Autodesk Inventor part; units mm, degrees
ref_plane "YZ Plane" through (0, 0, 0) normal (1, 0, 0) x (0, 1, 0)
ref_plane "XZ Plane" through (0, 0, 0) normal (0, 1, 0) x (-1, 0, 0)
ref_plane "XY Plane" through (0, 0, 0) normal (0, 0, 1) x (1, 0, 0)
sketch "Sketch1" plane through (0, 0, 0) normal (0, 1, 0) x (-1, 0, 0)
  line L0 (85, 50) -> (-85, 50)
  line L1 (-85, 50) -> (-85, -50)
  line L2 (-85, -50) -> (85, -50)
  line L3 (85, -50) -> (85, 50)
  line L4 (85, 50) -> (-85, -50) construction
  line L5 (-85, 50) -> (85, -50) construction
  point P0 (0, 0)
  dimension "d0" = 170
  dimension "d1" = 100
extrude "Extrusion1" add sketch "Sketch1" along normal blind 3.125
sketch "Sketch2" plane through (0, 3.125, 0) normal (0, 1, 0) x (1, 0, 0)
  line L0 (-26.702, 10) -> (-6.702, 10)
  line L1 (-6.702, 10) -> (-6.702, -10)
  line L2 (-6.702, -10) -> (-26.702, -10)
  line L3 (-26.702, -10) -> (-26.702, 10)
  line L4 (-26.702, 10) -> (-6.702, -10) construction
  line L5 (-6.702, 10) -> (-26.702, -10) construction
  circle A0 centre (-16.702, 0) radius 7.5
  line L6 (25.8262, 10) -> (45.8262, 10)
  line L7 (45.8262, 10) -> (45.8262, -10)
  line L8 (45.8262, -10) -> (25.8262, -10)
  line L9 (25.8262, -10) -> (25.8262, 10)
  line L10 (25.8262, 10) -> (45.8262, -10) construction
  line L11 (45.8262, 10) -> (25.8262, -10) construction
  circle A1 centre (35.8262, 0) radius 7.5
  line L12 (0.1504, 0) -> (2.6516, 0) construction
  point P0 (0, 0)
  dimension "d13" = 0
  dimension "d4" = 20
  dimension "d5" = 20
  dimension "d6" = 15
  dimension "d14" = 20
  dimension "d15" = 20
  dimension "d16" = 15
extrude "Extrusion2" add sketch "Sketch2" along normal blind 22.4 contours A0 | A1
extrude "Extrusion3" add sketch "Sketch2" along normal blind 10 contours L0 L1 L2 L3 | L6 L7 L8 L9 | A1
sketch "Sketch3" plane through (-16.702, 25.525, 0) normal (0, 1, 0) x (1, 0, 0)
  circle A0 centre (0, 0) radius 3
  point P0 (16.702, 0)
  dimension "d11" = 6
extrude "Extrusion4" cut sketch "Sketch3" against normal blind 7
sketch "Sketch4" plane through (35.8262, 25.525, 0) normal (0, 1, 0) x (1, 0, 0)
  circle A0 centre (0, 0) radius 3
  point P0 (-35.8262, 0)
  dimension "d17" = 6
extrude "Extrusion5" cut sketch "Sketch4" against normal blind 7
sketch "Sketch5" plane through (0, 3.125, 0) normal (0, 1, 0) x (1, 0, 0)
  line L0 (85, 50) -> (-85, 50)
  line L1 (-85, 50) -> (85, 50)
  line L2 (85, 50) -> (85, 51.3)
  line L3 (85, 51.3) -> (-85, 51.3)
  line L4 (-85, 51.3) -> (-85, 50)
  line L5 (-85, -50) -> (85, -50)
  line L6 (-85, -50) -> (85, -50)
  line L7 (85, -50) -> (85, -51.3)
  line L8 (85, -51.3) -> (-85, -51.3)
  line L9 (-85, -51.3) -> (-85, -50)
  line L10 (85, -51.3) -> (87, -51.3)
  line L11 (87, -51.3) -> (87, 51.3)
  line L12 (87, 51.3) -> (85, 51.3)
  line L13 (85, 51.3) -> (85, -51.3)
  point P0 (0, 0)
  point P1 (85, -50)
  dimension "d20" = 1.3
  dimension "d21" = 1.3
  dimension "d22" = 2
extrude "Extrusion6" add sketch "Sketch5" along normal blind 25.525
sketch "Sketch6" plane through (-85, 0, 50) normal (0, 0, 1) x (1, 0, 0)
  line L0 (170, 0) -> (0, 0)
  line L1 (170, 0) -> (170, 3.125)
  line L2 (0, 0) -> (170, 0)
  line L3 (170, 0) -> (170, 3.125)
  line L4 (170, 3.125) -> (0, 3.125)
  line L5 (0, 3.125) -> (0, 0)
  point P0 (85, 0)
extrude "Extrusion7" add sketch "Sketch6" along normal blind 1.3
sketch "Sketch7" plane through (85, 0, -50) normal (0, 0, -1) x (-1, 0, 0)
  line L0 (0, 0) -> (0, 3.125)
  line L1 (170, 0) -> (170, 28.65)
  line L2 (0, 0) -> (170, 0)
  line L3 (170, 0) -> (170, 2.2028)
  line L4 (170, 2.2028) -> (0, 2.2028)
  line L5 (0, 2.2028) -> (0, 0)
extrude "Extrusion8" add sketch "Sketch7" along normal blind 1.3
sketch "Sketch8" plane through (85, 0, 51.3) normal (1, 0, 0) x (0, 0, -1)
  line L0 (0, 0) -> (0, 3.125)
  line L1 (0, 0) -> (102.6, 0)
  line L2 (0, 3.125) -> (102.6, 3.125)
  line L3 (102.6, 3.125) -> (102.6, 0)
  line L4 (102.6, 0) -> (0, 0)
  line L5 (0, 0) -> (0, 3.125)
  point P0 (51.3, 0)
extrude "Extrusion9" add sketch "Sketch8" along normal blind 2
sketch "Sketch9" plane through (0, 3.125, 0) normal (0, 1, 0) x (1, 0, 0)
  line L0 (85, -50) -> (85, 50)
  line L1 (85, 50) -> (65, 50)
  line L2 (65, 50) -> (65, 45)
  line L3 (65, 45) -> (85, 45)
  line L4 (85, 45) -> (85, 50)
  line L5 (85, -50) -> (65, -50)
  line L6 (65, -50) -> (65, -45)
  line L7 (65, -45) -> (85, -45)
  line L8 (85, -45) -> (85, -50)
  point P0 (0, 0)
  dimension "d31" = 20
  dimension "d32" = 5
  dimension "d33" = 20
  dimension "d34" = 5
extrude "Extrusion10" add sketch "Sketch9" along normal blind 22.4
sketch "Sketch10" plane through (-85, 3.125, 50) normal (0, 0, -1) x (-1, 0, 0)
  line L0 (-170, 25.525) -> (0, 25.525)
  line L1 (-143.8389, 3.6428) -> (-91.9175, 3.6428)
  line L2 (-91.9175, 3.6428) -> (-91.9175, 25.525)
  line L3 (-91.9175, 25.525) -> (-143.8389, 25.525)
  line L4 (-143.8389, 25.525) -> (-143.8389, 3.6428)
  point P0 (-150, 27.4)
  point P1 (-143.8389, 25.525)
extrude "Extrusion11" cut sketch "Sketch10" against normal blind 27.4
mirror "Mirror1" about plane through (0, 0, 0) normal (0, 0, 1) of "Extrusion11"
sketch "Sketch11" plane through (0, 3.125, 0) normal (0, 1, 0) x (1, 0, 0)
  line L0 (47.3531, -30.5) -> (27.3531, -30.5)
  line L1 (27.3531, -30.5) -> (27.3531, -23.5)
  line L2 (27.3531, -23.5) -> (47.3531, -23.5)
  line L3 (47.3531, -23.5) -> (47.3531, -30.5)
  line L4 (-85, -50) -> (65, -50)
  point P0 (0, 0)
  dimension "d39" = 7
  dimension "d42" = 19.5
  dimension "d43" = 20
extrude "Extrusion12" add sketch "Sketch11" along normal blind 15
sketch "Sketch12" plane through (0, 3.125, 0) normal (0, 1, 0) x (1, 0, 0)
  line L0 (27.3531, -23.5) -> (47.3531, -23.5)
  line L1 (47.3531, -23.5) -> (27.3531, -23.5)
  line L2 (27.3531, -23.5) -> (27.3531, -21.5)
  line L3 (27.3531, -21.5) -> (47.3531, -21.5)
  line L4 (47.3531, -21.5) -> (47.3531, -23.5)
  point P0 (0, 0)
  dimension "d44" = 2
extrude "Extrusion13" add sketch "Sketch12" along normal blind 3
mirror "Mirror2" about plane through (0, 0, 0) normal (0, 0, 1) of "Extrusion12", "Extrusion13"
sketch "Sketch13" plane through (0, 3.125, 0) normal (0, 1, 0) x (1, 0, 0)
  line L0 (-85, -50) -> (65, -50)
  line L1 (6.5534, -50) -> (3.5534, -50)
  line L2 (3.5534, -50) -> (3.5534, -38)
  line L3 (3.5534, -38) -> (6.5534, -38)
  line L4 (6.5534, -38) -> (6.5534, -50)
  point P0 (0, 0)
  dimension "d47" = 3
  dimension "d48" = 12
extrude "Extrusion14" add sketch "Sketch13" along normal blind 6
mirror "Mirror3" about plane through (0, 0, 0) normal (0, 0, 1) of "Extrusion14"
sketch "Sketch14" plane through (0, 3.125, 0) normal (0, 1, 0) x (1, 0, 0)
  line L0 (-85, -50) -> (3.5534, -50)
  line L1 (-6.3506, -50) -> (-26.3506, -50)
  line L2 (-26.3506, -50) -> (-26.3506, -45)
  line L3 (-26.3506, -45) -> (-6.3506, -45)
  line L4 (-6.3506, -45) -> (-6.3506, -50)
  point P0 (0, 0)
  dimension "d51" = 20
  dimension "d52" = 5
extrude "Extrusion15" add sketch "Sketch14" along normal blind 20
mirror "Mirror4" about plane through (0, 0, 0) normal (0, 0, 1) of "Extrusion15"
sketch "Sketch15" plane through (-85, 3.125, 50) normal (0, 0, -1) x (-1, 0, 0)
  line L0 (0, 0) -> (-58.6494, 0)
  line L1 (-91.9175, 25.525) -> (0, 25.525)
  line L2 (0, 0) -> (-30.3469, 0)
  line L3 (-30.3469, 0) -> (-30.3469, 25.525)
  line L4 (-30.3469, 25.525) -> (0, 25.525)
  line L5 (0, 25.525) -> (0, 0)
  point P0 (-85, -3.125)
  point P1 (0, 25.525)
  point P2 (-30.3469, 0)
extrude "Extrusion16" cut sketch "Sketch15" against normal blind 20
mirror "Mirror5" about plane through (0, 0, 0) normal (0, 0, 1) of "Extrusion16"
sketch "Sketch17" plane through (-85, 2.2028, -50) normal (0, 1, 0) x (1, 0, 0)
  line L0 (170, 0) -> (0, 0)
  line L1 (0, 0) -> (170, 0)
  line L2 (170, 0) -> (170, 1.3)
  line L3 (170, 1.3) -> (0, 1.3)
  line L4 (0, 1.3) -> (0, 0)
  point P0 (85, -50)
extrude "Extrusion19" add sketch "Sketch17" along normal blind 0.922
sketch "Sketch18" plane through (0, 28.65, 0) normal (0, 1, 0) x (1, 0, 0)
  line L0 (85, 51.3) -> (-85, 51.3)
  line L1 (-85, -51.3) -> (87, -51.3)
  line L2 (-85, 51.3) -> (-50.9649, 51.3)
  line L3 (-50.9649, 51.3) -> (-50.9649, -51.3)
  line L4 (-50.9649, -51.3) -> (-85, -51.3)
  line L5 (-85, -51.3) -> (-85, 51.3)
  point P0 (0, 0)
extrude "Extrusion20" cut sketch "Sketch18" against normal blind 125.922
sketch "Sketch24" plane through (-26.3506, 3.125, 45) normal (-1, 0, 0) x (0, 0, 1)
  line L0 (0, 20) -> (5, 20)
  line L1 (5, 0) -> (0, 0)
  line L2 (0, 0) -> (0, 20)
  line L3 (0, 20) -> (5, 20)
  line L4 (5, 20) -> (5, 0)
  point P0 (-45, -3.125)
extrude "Extrusion26" add sketch "Sketch24" along normal blind 19.25
sketch "Sketch25" plane through (-26.3506, 3.125, -45) normal (-1, 0, 0) x (0, 0, 1)
  line L0 (-5, 0) -> (-5, 20)
  line L1 (-5, 0) -> (0, 0)
  line L2 (0, 0) -> (0, 20)
  line L3 (0, 20) -> (-5, 20)
  line L4 (-5, 20) -> (-5, 0)
  point P0 (45, -3.125)
extrude "Extrusion27" add sketch "Sketch25" along normal blind 19.25
sketch "Sketch26" plane through (87, 0, 51.3) normal (0, 0, 1) x (1, 0, 0)
  line L0 (-137.9649, 0) -> (0, 0)
  line L1 (-137.9649, 0) -> (-116.6587, 0)
  line L2 (-116.6587, 0) -> (-116.6587, 28.65)
  line L3 (-137.9649, 28.65) -> (-80.0825, 28.65)
  line L4 (-116.6587, 28.65) -> (-137.9649, 0)
  line L5 (-137.9649, 28.65) -> (-137.9649, 3.125)
  line L6 (-116.6587, 28.65) -> (-137.9649, 28.65)
  line L7 (-137.9649, 28.65) -> (-137.9649, 0)
  point P0 (-87, 0)
  point P1 (-137.9649, 3.125)
extrude "Extrusion28" cut sketch "Sketch26" against normal blind 133 contours L7 L5 L3 L4
sketch "Sketch29" plane through (87, 0, -51.3) normal (0, 0, -1) x (-1, 0, 0)
  line L0 (0, 0) -> (0, 28.65)
  line L1 (28.1611, 28.65) -> (0, 28.65)
  line L2 (0, 0) -> (0, 28.65)
  line L3 (28.1611, 28.65) -> (28.1611, 6.7678)
  line L4 (0, 28.65) -> (28.1611, 28.65)
  line L5 (28.1611, 28.65) -> (28.1611, 6.7678)
  line L6 (80.4466, 3.125) -> (80.4466, 9.125)
  line L7 (28.1611, 6.7678) -> (80.0825, 6.7678)
  line L8 (80.0825, 6.7678) -> (28.1611, 6.7678)
  line L9 (116.6587, 28.65) -> (80.0825, 28.65)
  line L10 (80.0825, 6.7678) -> (80.0825, 28.65)
  line L11 (80.0825, 28.65) -> (116.6587, 28.65)
  line L12 (116.6587, 28.65) -> (137.9649, 0)
  line L13 (116.6587, 28.65) -> (137.9649, 0)
  line L14 (137.9649, 0) -> (0, 0)
  point P0 (87, 0)
extrude "Extrusion31" add sketch "Sketch29" along normal blind 0.5
mirror "Mirror6" about plane through (0, 0, 0) normal (0, 0, 1) of "Extrusion31"
properties part number "Sujeta_motor_3DPrint"
Source: CAD feature listing. Evaluate the final solid. Frame: model axes, mm. A direction names the side the tool comes from. Give positions to 0.01 mm unless a question says otherwise; leave off trailing zeros. Loops run counter-clockwise (first coordinate to the right, second up) from the corner with the lowest first, then second, coordinate; pieces in that order, holes last. Notation, with made-up numbers: (50, 7) - (87, 7) arc R28 ccw to (87, 40) - close; hole circle Ø7 at (57, -22). An arc over 180 degrees is marked (long way). Use CSV: the item, a comma, the result in double quotes. Start each with the question number.
1. Section A-A (y = 20). Output: boundary loops of the cut face in (x, z).
2. Ray query, L1, parallel to X at y = 20, z = 0; L2, parallel to Z at x = 3, y = 4; L3, parallel to Z at x = -14.5, y = 13.75. Return the intervals inside material, ascending.
3. Reachability of faces 4 (the flat face through (-20, 23.125, -47)), 5 (the flat face through (39, 25.525, 0)), 6 (the flat face through (75, 14, 45)) from +Z, -Z, +X, -X, +Y, -Y: full face, straight path, thin tool, end or side. Return the list, or none.
4. Pin query (flat end, axial travel): pin 1 (10 mm diameter, centred on y = 12.5, z = 26, fed in from -X); pin 2 (3.5 mm diameter, centred on x = -48, y = 6, fed in from -Z); pin 3 (6 mm diameter, centred on x = 34.5, z = -5, fed in from +Y) (3 decimals); pin 4 (1 mm diameter, centred on y = 23, z = -13.5, fed in from -X). Return the tip coordinate at first contact, or that it passes through.
5. Draft query along Z for faces 1 (the flat face through (19, 0, -1)), 2 (the flat face through (37, 5, -21.5)), 3 (the flat face through (17, 5, 51.8)). Return one class per face: +Z half, -Z half, draft (parallel to the pull), parting line (faces both ways), or undercut.
Response:
1,outline,"(-36.09, -51.8) - (6.92, -51.8) - (6.92, -50) - (-6.35, -50) - (-6.35, -45) - (-36.09, -45) - close; (-36.09, 45) - (-6.35, 45) - (-6.35, 50) - (6.92, 50) - (6.92, 51.8) - (-36.09, 51.8) - close; circle Ø15 at (-16.7, 0); circle Ø15 at (35.83, 0); (58.84, -51.8) - (87, -51.8) - (87, 51.8) - (58.84, 51.8) - (58.84, 50) - (65, 50) - (65, 45) - (85, 45) - (85, -45) - (65, -45) - (65, -50) - (58.84, -50) - close; hole circle Ø6 at (-16.7, 0); hole circle Ø6 at (35.83, 0)"
2,L1,"-24.2 to -19.7, -13.7 to -9.2, 28.33 to 32.83, 38.83 to 43.33, 85 to 87"
2,L2,"-51.8 to -50, 50 to 51.8"
2,L3,"-51.8 to -45, -7.17 to 7.17, 45 to 51.8"
3,face 4,"-X, +Y"
3,face 5,"+Z, -Z, -X, +Y"
3,face 6,"+Y"
4,pin 1,"x = 27.35"
4,pin 2,"z = -51.8"
4,pin 3,"y = 25.525"
4,pin 4,"x = 85"
5,face 1,"draft"
5,face 2,"undercut"
5,face 3,"+Z half"
